For this review, take the finished solid that the model builds, in its own axes (mm). A direction names the side the tool comes from. Coordinates: 2 decimals unless noted, no trailing zeros. Loops run counter-clockwise (first coordinate to the right, second up) from the corner with the lowest first, then second, coordinate; pieces in that order, holes last. Notation, with made-up numbers: (88, 5) -> (104, 5) arc R32 cw to (104, 32) -> close; hole circle Ø2 at (51, 59). An arc over 180 degrees is marked (long way). Answer in a Markdown table with one row per item.
from build123d import *

# Parameters (mm, degrees)
SKETCH1_R      = 4.25
EXTRUDE1_DEPTH = 1.25


with BuildPart() as part:
    # Sketch1 → Extrude1 (new body, symmetric)
    with BuildSketch(Plane.XY):
        with BuildLine():
            Line((11, 0), (11, 18.718207384))
            ThreePointArc((11, 18.718207384), (10.980438994, 18.997243926), (10.922138608, 19.270822234))
            Line((10.922138608, 19.270822234), (8.541123231, 27.55261485))
            ThreePointArc((8.541123231, 27.55261485), (7.822057834, 28.597690474), (6.618984623, 29))
            Line((6.618984623, 29), (5.125, 29))
            ThreePointArc((5.125, 29), (4.417893219, 28.707106781), (4.125, 28))
            Line((4.125, 28), (4.125, 19.5))
            ThreePointArc((4.125, 19.5), (3.978553391, 19.146446609), (3.625, 19))
            Line((3.625, 19), (-3.625, 19))
            ThreePointArc((-3.625, 19), (-3.978553391, 19.146446609), (-4.125, 19.5))
            Line((-4.125, 19.5), (-4.125, 28))
            ThreePointArc((-4.125, 28), (-4.417893219, 28.707106781), (-5.125, 29))
            Line((-5.125, 29), (-6.618984623, 29))
            ThreePointArc((-6.618984623, 29), (-7.822057834, 28.597690474), (-8.541123231, 27.55261485))
            Line((-8.541123231, 27.55261485), (-10.922138608, 19.270822234))
            ThreePointArc((-10.922138608, 19.270822234), (-10.980438994, 18.997243926), (-11, 18.718207384))
            Line((-11, 18.718207384), (-11, 0))
            ThreePointArc((-11, 0), (0, -11), (11, 0))
        make_face()
        Circle(SKETCH1_R, mode=Mode.SUBTRACT)
    extrude(amount=EXTRUDE1_DEPTH, both=True)


solid = part.part
Item 1: Insertion check: pin 1 (1.2 mm diameter, centred on x = 0, z = -0.5, fed in from +Y); pin 2 (10 mm diameter, centred on x = 0, y = 0, fed in from +Z); pin 3 (1.2 mm diameter, centred on y = 22.5, z = 0.5, fed in from -X); pin 4 (1.2 mm diameter, centred on y = 22, z = -0.5, fed in from +X). Each pin has a flat end and moves straight along its axis. Give the tip position at first contact, or say it passes through.
Worked answers:
| item | result |
|---|---|
| pin 1 | y = 19 |
| pin 2 | z = 1.25 |
| pin 3 | x = -10.17 |
| pin 4 | x = 10.31 |
Item 2: Take a section at A-A, the plane x = 0. State the section outline as (y, z) points, and give its area (4 significant figures).
Worked answers:
| item | result |
|---|---|
| outline | (-11, -1.25) -> (-4.25, -1.25) -> (-4.25, 1.25) -> (-11, 1.25) -> close; (4.25, -1.25) -> (19, -1.25) -> (19, 1.25) -> (4.25, 1.25) -> close |
| area | 53.75 mm² |
Item 3: Take a section at C-C, the plane z = -0.3. State the section outline as (x, y) points (3 decimals), and give its area (3 significant figures).
Worked answers:
| item | result |
|---|---|
| outline | (-11, 0) arc R11 ccw to (11, 0) -> (11, 18.718) arc R2 ccw to (10.922, 19.271) -> (8.541, 27.553) arc R2 ccw to (6.619, 29) -> (5.125, 29) arc R1 ccw to (4.125, 28) -> (4.125, 19.5) arc R0.5 cw to (3.625, 19) -> (-3.625, 19) arc R0.5 cw to (-4.125, 19.5) -> (-4.125, 28) arc R1 ccw to (-5.125, 29) -> (-6.619, 29) arc R2 ccw to (-8.541, 27.553) -> (-10.922, 19.271) arc R2 ccw to (-11, 18.718) -> close; hole circle Ø8.5 at (0, 0) |
| area | 659 mm² |
Item 4: For faces 1 (the cylindrical face through (0, -11, 0)), 2 (the flat face through (4.125, 24, 0)), list the 3-axis set-ups (+Z, -Z, +X, -X, +Y, -Y) from which the entire face can be reached by the end or side of a thin tool; tool diameter is ignored.
Worked answers:
| item | result |
|---|---|
| face 1 | +Z, -Z, -Y |
| face 2 | +Z, -Z, +Y |
Item 5: The part is to be moulded in two halves that separate along X. For faces 3 (the cylindrical face through (2.285, 3.584, -0.018)), 4 (the cylindrical face through (7.836, 28.587, 0.018)), 5 (the flat face through (-9.715, 23.47, 0.018)), 6 (the flat face through (-4.125, 24, 0)), say which applies: +X half, -X half, draft (parallel to the pull), parting line (faces both ways), or undercut.
Worked answers:
| item | result |
|---|---|
| face 3 | undercut |
| face 4 | +X half |
| face 5 | -X half |
| face 6 | undercut |
Item 6: Take a section at B-B, the plane y = 21. State the section outline as (x, z) points (3 decimals).
Worked answers:
| item | result |
|---|---|
| outline | (-10.425, -1.25) -> (-4.125, -1.25) -> (-4.125, 1.25) -> (-10.425, 1.25) -> close; (4.125, -1.25) -> (10.425, -1.25) -> (10.425, 1.25) -> (4.125, 1.25) -> close |
Item 7: For L1, parallel to Y at x = 0, z = -0.2; L2, parallel to Y at x = -2.25, z = 0.7; L3, parallel to X at y = 25, z = -1.1 (3 decimals), list the stretches that pass through material, from the lowest coordinate up.
Worked answers:
| item | result |
|---|---|
| L1 | -11 to -4.25, 4.25 to 19 |
| L2 | -10.77 to -3.61, 3.61 to 19 |
| L3 | -9.275 to -4.125, 4.125 to 9.275 |
